Geometry: see drawing. Coordinates: mm, zero at the bounding-box minimum. A direction names the side the tool comes from. Coordinates: 2 decimals unless noted, no trailing zeros. Write each loop counter-clockwise with the first axis right and the second up, starting at its lowest first coordinate (ties: lowest second). Pieces come first, ordered by that corner, then holes. Notation, with made-up numbers: M 46.5,36 L 64.5,36 A9 ccw 64.5,50 Z; hole C 58,2 d11. An arc over 180 degrees is marked long. One line per item, written item: value. Start each with the question number.
Item 1: Set-up query: the marked faces 1 and 2. Return all of +Z, -Z, +X, -X, +Y, -Y with unobstructed straight access to the full face (end or side cutting, diameter ignored); none if empty.
Item 2: Cut plane C-C, the plane y = 1. Output: boundary loops of the cut face in (x, z), then the cut area to 3 significant figures.
Item 3: Cut plane D-D, the plane x = 7.5. Output: boundary loops of the cut face in (y, z).
Item 4: Cut plane A-A, the plane y = 8.5. State how many separate pieces and enclosed holes the cut face has, then the cut area to 3 significant figures.
Item 5: Pin query (flat end, axial travel): P1, Ø1.5, axis at x = 15.75, z = 15.75, coming from the +Y side; P2, Ø5.5, axis at x = 7, z = 31, coming from the +Y side; P3, Ø3, axis at x = 52.5, y = 11, coming from the -Z side. Return the tip coordinate at first contact, or that it passes through.
Item 6: Ray query, L1, parallel to X at y = 9.5, z = 31.75; L2, parallel to Z at x = 29, y = 10.25; L3, parallel to Y at x = 51, z = 51. Return the intervals inside material, ascending. Write a range as from..to.
Item 7: Cut plane B-B, the plane x = 31.75. Output: boundary loops of the cut face in (y, z), then the cut area to 3 significant figures.
Item 8: Mould query, pull axis Z, two halves, no side actions, for the marked faces 3, 4 and 5. Classes: released by +Z, released by -Z, zero draft, split by the parting line, or undercut.
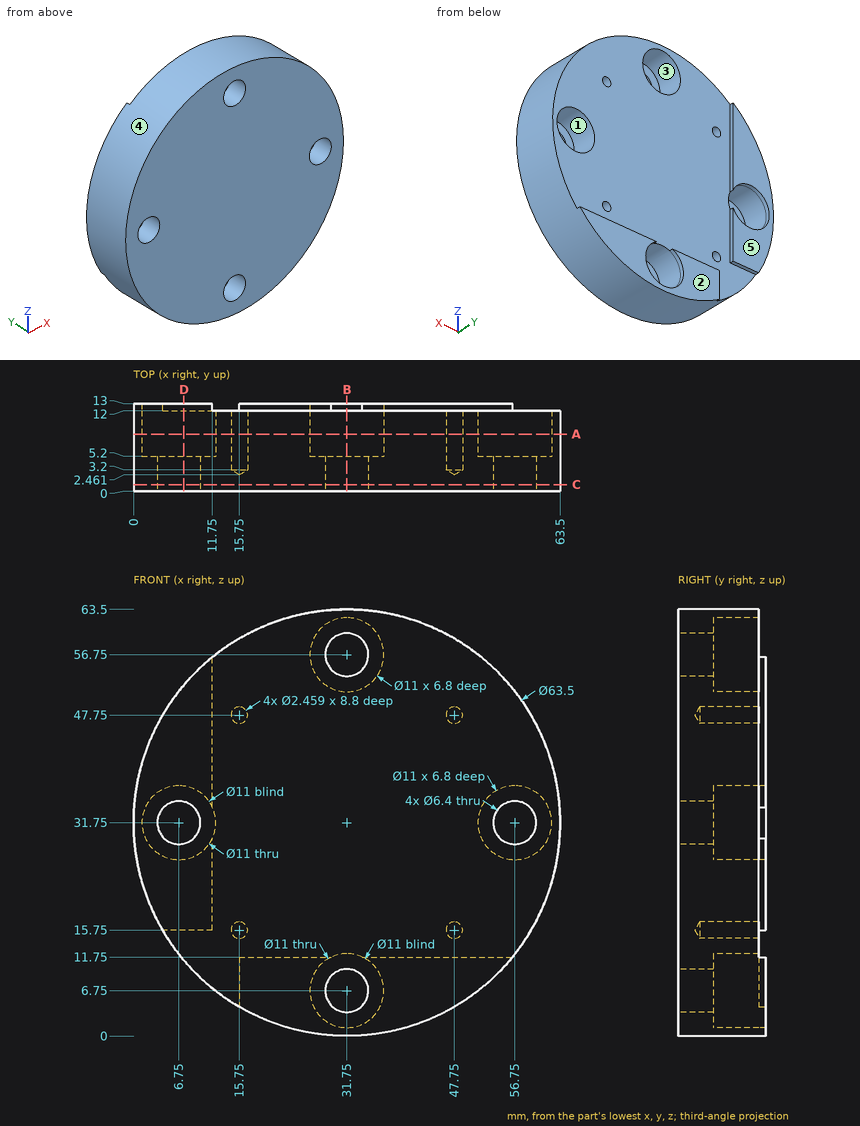
From the geometry:
1. face 1: +Y
1. face 2: +Z, -Z, +X, -X, +Y
2. outline: C 31.75,31.75 d63.5; hole C 6.75,31.75 d6.4; hole C 31.75,6.75 d6.4; hole C 31.75,56.75 d6.4; hole C 56.75,31.75 d6.4
2. area: 3,040 mm²
3. outline: M 0,11.26 L 12,11.26 L 12,15.75 L 13,15.75 L 13,26.3 L 5.2,26.3 L 5.2,28.64 L 0,28.64 Z; M 0,34.86 L 5.2,34.86 L 5.2,37.2 L 13,37.2 L 13,52.24 L 0,52.24 Z
4. separate pieces: 1
4. enclosed holes: 8
4. area: 2,770 mm²
5. P1: stops at y = 2.91
5. P2: stops at y = 5.2
5. P3: stops at z = 6.5
6. L1: x = 0..1.25, 12.25..51.25, 62.25..63.5
6. L2: z = 0.12..1.99, 11.51..51.99, 61.51..63.38
6. L3: y = 0..12
7. outline: M 0,0 L 13,0 L 13,1.25 L 5.2,1.25 L 5.2,3.55 L 0,3.55 Z; M 0,9.95 L 5.2,9.95 L 5.2,12.25 L 12,12.25 L 12,51.25 L 5.2,51.25 L 5.2,53.55 L 0,53.55 Z; M 0,59.95 L 5.2,59.95 L 5.2,62.25 L 12,62.25 L 12,63.5 L 0,63.5 Z
7. area: 547 mm²
8. face 3: undercut
8. face 4: split by the parting line
8. face 5: zero draft
